Autodesk Inventor part; units mm, degrees
ref_plane "to_bearings_XY" through (14, 0, 0) normal (1, 0, 0) x (0, 0, -1)
ref_plane "to_bearings_YZ" through (14, 0, 0) normal (0, 0, -1) x (0, 1, 0)
ref_plane "to_bearings_ZX" through (14, 0, 0) normal (0, 1, 0) x (1, 0, 0)
sketch "Sketch_1" plane through (0, 0, 0) normal (0, 0, 1) x (1, 0, 0)
  line L0 (22, 0) -> (0, 0)
  line L1 (0, 30) -> (0, 12)
  line L2 (0, 12) -> (14, 12)
  line L3 (14, 12) -> (14, 15.5)
  line L4 (14, 15.5) -> (22, 15.5)
  line L5 (22, 15.5) -> (22, 30)
  line L6 (22, 30) -> (0, 30)
revolve "Revolution1" add sketch "Sketch_1" angle 360 about axis through (22, 0, 0) along (1, 0, 0)
sketch "Sketch_2" plane through (0, 0, 0) normal (1, 0, 0) x (0, 1, 0)
  line L0 (-120, 80) -> (-120, -80)
  line L1 (-120, -80) -> (120, -80)
  line L2 (120, -80) -> (120, 80)
  line L3 (120, 80) -> (-120, 80)
  line L4 (-30, 20) -> (-30, -20)
  line L5 (-30, -20) -> (30, -20)
  line L6 (30, -20) -> (30, 20)
  line L7 (30, 20) -> (-30, 20)
extrude "Extrusion1" cut sketch "Sketch_2" along normal blind 24
sketch "Sketch_3" plane through (0, 0, 0) normal (0, 0, 1) x (1, 0, 0)
  line L0 (22, 23) -> (0, 23)
  line L1 (0, 23) -> (0, 27)
  line L2 (0, 27) -> (0.6765, 26.3235)
  line L3 (0.6765, 26.3235) -> (14.8235, 26.3235)
  line L4 (14.8235, 26.3235) -> (15.5, 27)
  line L5 (15.5, 27) -> (15.5, 28.5)
  line L6 (15.5, 28.5) -> (22, 28.5)
  line L7 (22, 28.5) -> (22, 23)
  line L8 (22, 23) -> (0, 23)
revolve "Revolution2" cut sketch "Sketch_3" angle 360 about axis through (22, 23, 0) along (1, 0, 0)
thread "Thread1"
pattern_linear "Rectangular Pattern1" count 2 spacing 46 along (0, -1, 0) of "Revolution2"
sketch "Sketch_4" plane through (7.5, 0, 0) normal (1, 0, 0) x (0, 0, -1)
  line L0 (-11.65, 0) -> (-20, 0)
  line L1 (-20, 0) -> (-20, 2.5)
  line L2 (-20, 2.5) -> (-19.567, 2.067)
  line L3 (-19.567, 2.067) -> (-12.083, 2.067)
  line L4 (-12.083, 2.067) -> (-11.65, 2.5)
  line L5 (-11.65, 2.5) -> (-11.65, 0)
  line L6 (-11.65, 0) -> (-20, 0)
revolve "Revolution3" cut sketch "Sketch_4" angle 360 about axis through (7.5, 0, 11.65) along (0, 0, -1)
thread "Thread2"
sketch "Sketch_6" plane through (7.5, 0, 0) normal (1, 0, 0) x (0, 0, -1)
  line L0 (20, 0) -> (11.65, 0)
  line L1 (11.65, 0) -> (11.65, 2.5)
  line L2 (11.65, 2.5) -> (12.083, 2.067)
  line L3 (12.083, 2.067) -> (19.567, 2.067)
  line L4 (19.567, 2.067) -> (20, 2.5)
  line L5 (20, 2.5) -> (20, 0)
  line L6 (20, 0) -> (11.65, 0)
revolve "Revolution4" cut sketch "Sketch_6" angle 360 about axis through (7.5, 0, -20) along (0, 0, -1)
thread "Thread3"
ref_plane "to_bearings_XY" through (14, 0, 0) normal (1, 0, 0) x (0, 0, -1)
ref_plane "to_bearings_YZ" through (14, 0, 0) normal (0, 0, -1) x (0, 1, 0)
ref_plane "to_bearings_ZX" through (14, 0, 0) normal (0, 1, 0) x (1, 0, 0)
ref_plane "to_screw1_XY" through (7.5, 0, 12) normal (0, 0, 1) x (1, 0, 0)
ref_plane "to_screw1_YZ" through (7.5, 0, 12) normal (1, 0, 0) x (0, 1, 0)
ref_plane "to_screw1_ZX" through (7.5, 0, 12) normal (0, 1, 0) x (0, 0, 1)
ref_plane "to_screw2_XY" through (7.5, 0, -12) normal (0, 0, -1) x (1, 0, 0)
ref_plane "to_screw2_YZ" through (7.5, 0, -12) normal (1, 0, 0) x (0, -1, 0)
ref_plane "to_screw2_ZX" through (7.5, 0, -12) normal (0, -1, 0) x (0, 0, -1)
properties part number "BGCSB12_h"
Work out the finished part from the listing and answer in its coordinate system (mm). A direction names the side the tool comes from. Coordinates: 2 decimals unless noted, no trailing zeros. Loops run counter-clockwise (first coordinate to the right, second up) from the corner with the lowest first, then second, coordinate; pieces in that order, holes last. Notation, with made-up numbers: (-29.75, 41) - (6.25, 41) arc R32 cw to (6.25, 70) - close; hole circle Ø4 at (71, 79.25). An arc over 180 degrees is marked (long way). Use a Markdown table: item, result.
Item 1: Find section C-C, the plane z = 0. State how many separate pieces and enclosed holes the cut face has, and give its area (3 significant figures).
Evaluation:
| item | result |
|---|---|
| separate pieces | 4 |
| enclosed holes | 0 |
| area | 385 mm2 |
Item 2: Find section D-D, the plane y = 6.5. Determine the outline of the cut face in (x, z).
Evaluation:
| item | result |
|---|---|
| outline | (0, -20) - (22, -20) - (22, -14.07) - (14, -14.07) - (14, -10.09) - (0, -10.09) - close; (0, 10.09) - (14, 10.09) - (14, 14.07) - (22, 14.07) - (22, 20) - (0, 20) - close |
Item 3: Consider probe 1 along Z at (x, y) = (19, 0); probe 2 along Z at (x, y) = (3.75, 0); probe 3 along X at (y, z) = (0, 14). Determine where each line is inside the solid, lowest interval first. Write a range as from..to.
Evaluation:
| item | result |
|---|---|
| probe 1 | z = -20..-15.5, 15.5..20 |
| probe 2 | z = -20..-12, 12..20 |
| probe 3 | x = 0..5.43, 9.57..14 |
Item 4: Given pin 1 Ø10 at (x, z) = (3.5, 3.5) entering from +Y; pin 2 Ø8 at (x, z) = (15.5, -14) entering from -Y; pin 3 Ø10 at (y, z) = (-7.5, 3) entering from +X; pin 4 Ø3.5 at (x, y) = (7.5, 0) entering from +Z, each flat-ended and moving along its own axis, determine where each tip first touches the part or whether it passes through.
Evaluation:
| item | result |
|---|---|
| pin 1 | stops at y = 30 |
| pin 2 | stops at y = -28.28 |
| pin 3 | stops at x = 14 |
| pin 4 | passes through |
Item 5: Find section A-A, the plane y = 0. Determine the outline of the cut face in (x, z).
Evaluation:
| item | result |
|---|---|
| outline | (0, -20) - (5, -20) - (5.43, -19.57) - (5.43, -12.08) - (5.35, -12) - (0, -12) - close; (0, 12) - (5.35, 12) - (5.43, 12.08) - (5.43, 19.57) - (5, 20) - (0, 20) - close; (9.57, -19.57) - (10, -20) - (22, -20) - (22, -15.5) - (14, -15.5) - (14, -12) - (9.65, -12) - (9.57, -12.08) - close; (9.57, 12.08) - (9.65, 12) - (14, 12) - (14, 15.5) - (22, 15.5) - (22, 20) - (10, 20) - (9.57, 19.57) - close |
Item 6: For faces 1 (the flat face through (15.5, -27, -2)), 2 (the cylindrical face through (11, 30, 0)), determine the directions among +Z, -Z, +X, -X, +Y, -Y from which every point of the face is accessible in a straight line to the end or side of a thin tool.
Evaluation:
| item | result |
|---|---|
| face 1 | +X |
| face 2 | +X, -X, +Y |
Item 7: Find section B-B, the plane x = 7.5. Determine the outline of the cut face in (y, z), and give its area (3 significant figures).
Evaluation:
| item | result |
|---|---|
| outline | (-22.36, -20) - (-2.5, -20) - (-2.07, -19.57) - (-2.07, -12.08) - (-2.39, -11.76) arc R12 cw to (-2.39, 11.76) - (-2.07, 12.08) - (-2.07, 19.57) - (-2.5, 20) - (-22.36, 20) arc R30 ccw to start; (2.07, -19.57) - (2.5, -20) - (22.36, -20) arc R30 ccw to (22.36, 20) - (2.5, 20) - (2.07, 19.57) - (2.07, 12.08) - (2.39, 11.76) arc R12 cw to (2.39, -11.76) - (2.07, -12.08) - close; hole circle Ø6.65 at (-23, 0); hole circle Ø6.65 at (23, 0) |
| area | 1,620 mm2 |
Item 8: The mould has two halves that part along Z. Classify faces 3 (the flat face through (11, 0, 20)), 4 (the cylindrical face through (11, -30, 0)), 5 (the flat face through (14, 4.5, -11.4)): +Z half, -Z half, draft (parallel to the pull), parting line (faces both ways), or undercut.
Evaluation:
| item | result |
|---|---|
| face 3 | +Z half |
| face 4 | parting line |
| face 5 | undercut |
